```python
from build123d import *

# Parameters (mm, degrees)
IZIM1_W                     = 37.85
IZIM1_H                     = 25
IZIM1_R                     = 1.6
IZIM1_R_2                   = 4
Y_KSEKLIK_EKSTR_ZYON1_DEPTH = 2
IZIM2_W                     = 27.85
IZIM2_H                     = 2
Y_KSEKLIK_EKSTR_ZYON2_DEPTH = 2


with BuildPart() as part:
    # Çizim1 → Yükseklik-Ekstrüzyon1 (new body)
    with BuildSketch(Plane.XY):
        with Locations((7.675, 0)):
            Rectangle(IZIM1_W, IZIM1_H)
        with Locations((20.6, -8.75)):
            Circle(IZIM1_R, mode=Mode.SUBTRACT)
        with Locations((20.6, 8.75)):
            Circle(IZIM1_R, mode=Mode.SUBTRACT)
        Circle(IZIM1_R_2, mode=Mode.SUBTRACT)
    extrude(amount=Y_KSEKLIK_EKSTR_ZYON1_DEPTH)

    # Çizim2 → Yükseklik-Ekstrüzyon2 (add)
    with BuildSketch(Plane.XZ.offset(12.5)):
        with Locations((7.675, 1)):
            Rectangle(IZIM2_W, IZIM2_H)
    y_kseklik_ekstr_zyon2 = extrude(amount=Y_KSEKLIK_EKSTR_ZYON2_DEPTH)

    # Aynalama1: Yükseklik-Ekstrüzyon2 across plane
    add(y_kseklik_ekstr_zyon2.mirror(Plane.ZX))


solid = part.part
```
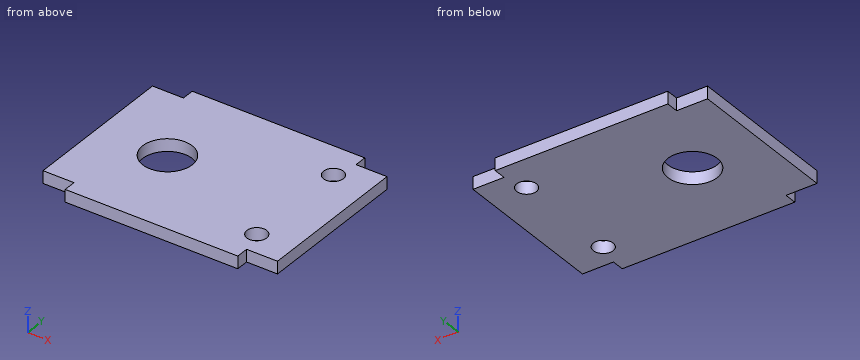
Here's how the part is built. I have some questions about the finished solid (model axes, mm). Coordinates: 2 decimals unless noted, no trailing zeros. Write each loop counter-clockwise with the first axis right and the second up, starting at its lowest first coordinate (ties: lowest second). Pieces come first, ordered by that corner, then holes. Notation, with made-up numbers: (88, 12.25) -> (100, 12.25) arc R16 cw to (100, 21.25) -> close; hole circle Ø11 at (54, 19). An arc over 180 degrees is marked (long way). Use a Markdown table: item, result. Add a question column.
(1) If we section it at D-D, the plane x = 20.6: Write out the boundary of the cut face in (y, z), and give its area (3 significant figures).
(2) If we section it at A-A, the plane x = 0: Write out the boundary of the cut face in (y, z), and give its area (3 significant figures).
(3) I'm going to push flat-ended pins straight in: P1, Ø0.6, axis at x = 23.5, z = 1.5, coming from the +Y side; P2, Ø0.6, axis at x = -9.5, z = 1, coming from the -Y side; P3, Ø1, axis at y = -13.5, z = 1.5, coming from the +X side; P4, Ø1.9, axis at x = 20.6, y = 8.75, coming from the +Z side. Where does each tip first touch, or does it pass through?
(4) Please list where these lines run through material, in increasing order: line 1 (Y direction, x = 20.6, z = 1.1); line 2 (Y direction, x = 0, z = 1.15); line 3 (Y direction, x = 21.5, z = 0.1).
(5) If we section it at C-C, the plane z = 1.5: Write out the boundary of the cut face in (x, y).
(6) If we section it at B-B, the plane y = 8.75: Write out the boundary of the cut face in (x, z), and give its area (3 significant figures).
Outcome:
| question | item | result |
|---|---|---|
| 1 | outline | (-14.5, 0) -> (-10.35, 0) -> (-10.35, 2) -> (-14.5, 2) -> close; (-7.15, 0) -> (7.15, 0) -> (7.15, 2) -> (-7.15, 2) -> close; (10.35, 0) -> (14.5, 0) -> (14.5, 2) -> (10.35, 2) -> close |
| 1 | area | 45.2 mm^2 |
| 2 | outline | (-14.5, 0) -> (-4, 0) -> (-4, 2) -> (-14.5, 2) -> close; (4, 0) -> (14.5, 0) -> (14.5, 2) -> (4, 2) -> close |
| 2 | area | 42.0 mm^2 |
| 3 | P1 | stops at y = 12.5 |
| 3 | P2 | stops at y = -12.5 |
| 3 | P3 | stops at x = 21.6 |
| 3 | P4 | passes through |
| 4 | line 1 | y = -14.5 to -10.35, -7.15 to 7.15, 10.35 to 14.5 |
| 4 | line 2 | y = -14.5 to -4, 4 to 14.5 |
| 4 | line 3 | y = -14.5 to -10.07, -7.43 to 7.43, 10.07 to 14.5 |
| 5 | outline | (-11.25, -12.5) -> (-6.25, -12.5) -> (-6.25, -14.5) -> (21.6, -14.5) -> (21.6, -12.5) -> (26.6, -12.5) -> (26.6, 12.5) -> (21.6, 12.5) -> (21.6, 14.5) -> (-6.25, 14.5) -> (-6.25, 12.5) -> (-11.25, 12.5) -> close; hole circle Ø8 at (0, 0); hole circle Ø3.2 at (20.6, -8.75); hole circle Ø3.2 at (20.6, 8.75) |
| 6 | outline | (-11.25, 0) -> (19, 0) -> (19, 2) -> (-11.25, 2) -> close; (22.2, 0) -> (26.6, 0) -> (26.6, 2) -> (22.2, 2) -> close |
| 6 | area | 69.3 mm^2 |
